Model file for the job. Use its own axes, mm. A direction names the side the tool comes from. Give positions to 0.01 mm unless a question says otherwise; leave off trailing zeros. Loops run counter-clockwise (first coordinate to the right, second up) from the corner with the lowest first, then second, coordinate; pieces in that order, holes last. Notation, with made-up numbers: M 16.25,67 L 49.25,67 A29 ccw 49.25,92 Z; hole C 71.25,61.25 d7. An arc over 180 degrees is marked long. Use CSV: the item, a comma, the result in double quotes. Start each with the question number.
(1) Tool access for faces 1 (the face through (-6.194, -24.694, 1.71)), 2 (the face through (-6, -12, 2)), 3 (the face through (-6.194, -0.306, 1.71)): list every direction of +Z, -Z, +X, -X, +Y, -Y with a clear straight run to the whole face (end or side of a thin tool).
(2) Slice it at A-A on z = 10.75. List the corners of the cut face in (x, y).
(3) Slice it at B-B on y = -6.5. List the corners of the cut face in (x, z), and give its area (3 significant figures).
(4) Wall check: line 1 along X through (y, z) = (-23.5, 4.5); line 2 along Z through (x, y) = (-2.75, -7.5); line 3 along Z through (x, y) = (-12, -18). Give the ranges that are in metal, low to high. Write a range as from..to.
(5) Flat gauge pins, fed straight in: P1, Ø4, axis at y = -15, z = 8, coming from the +X side; P2, Ø1, axis at x = -9, y = -4.5, coming from the +Z side; P3, Ø3, axis at x = -2, z = 5, coming from the +Y side; P4, Ø1.5, axis at x = -11.5, y = -19, coming from the -Z side. Where does each tip first touch, or does it go through?
(6) Slice it at C-C on x = -4. List the corners of the cut face in (y, z).
```python
from build123d import *

# Parameters (mm, degrees)
F1_DEPTH = 25
F2_R     = 1.016
F3_R     = 0.75
F4_R     = 0.762


with BuildPart() as f1:
    # F0 (on Front) → F1 (new body)
    with BuildSketch(Plane.XZ):
        with BuildLine():
            Line((-15, 0), (0, 0))
            Line((0, 0), (0, 2))
            Line((0, 2), (-11.476, 2))
            ThreePointArc((-11.476, 2), (-12.5536307345, 2.4463692655), (-13, 3.524))
            Line((-13, 3.524), (-13, 20))
            Line((-13, 20), (-15, 20))
            Line((-15, 20), (-15, 0))
        make_face()
    extrude(amount=F1_DEPTH)

    # F2
    f2_edges = [f1.edges().sort_by_distance(p)[0] for p in [
        (-13, -12.5, 3.524),
        (-13, -12.5, 20),
        (-13, 0, 11.762),
        (-13, -25, 11.762),
    ]]
    fillet(f2_edges, radius=F2_R)

    # F3
    f3_edges = [f1.edges().sort_by_distance(p)[0] for p in [
        (-15, 0, 10),
        (-15, -12.5, 20),
        (-15, -25, 10),
    ]]
    fillet(f3_edges, radius=F3_R)

    # F4
    f4_edges = [f1.edges().sort_by_distance(p)[0] for p in [
        (0, -25, 0.492),
        (0, -24.70242, 1.70242),
        (0, -12.5, 2),
        (0, -0.29758, 1.70242),
        (0, 0, 0.492),
    ]]
    fillet(f4_edges, radius=F4_R)


solid = f1.part
```
Reply:
1,face 1,"+Z, +X, -Y"
1,face 2,"+Z, +X, +Y, -Y"
1,face 3,"+Z, +X, +Y"
2,outline,"M -15,-24.25 A0.75 ccw -14.25,-25 L -14.02,-25 A1.02 ccw -13,-23.98 L -13,-1.02 A1.02 ccw -14.02,0 L -14.25,0 A0.75 ccw -15,-0.75 Z"
3,outline,"M -15,0 L 0,0 L 0,1.24 A0.76 ccw -0.76,2 L -11.48,2 A1.52 cw -13,3.52 L -13,18.98 A1.02 ccw -14.02,20 L -14.25,20 A0.75 ccw -15,19.25 Z"
3,area,"66.0 mm^2"
4,line 1,"x = -15..-13"
4,line 2,"z = 0..2"
4,line 3,"z = 0..2.09"
5,P1,"stops at x = -13"
5,P2,"stops at z = 2"
5,P3,"passes through"
5,P4,"stops at z = 0"
6,outline,"M -25,0 L 0,0 L 0,0.98 A1.02 ccw -1.02,2 L -23.98,2 A1.02 ccw -25,0.98 Z"
